For this review, take the finished solid that the model builds, in its own axes (mm). A direction names the side the tool comes from. Coordinates: 2 decimals unless noted, no trailing zeros. Loops run counter-clockwise (first coordinate to the right, second up) from the corner with the lowest first, then second, coordinate; pieces in that order, holes last. Notation, with made-up numbers: (-33.75, -14) - (11.25, -14) arc R21 cw to (11.25, 14) - close; hole circle Ø7 at (0, 20). An arc over 180 degrees is marked (long way). Use one line per item in the form item = value. Start each with the question number.
1. Add section C-C on x = 30. Give the boundary of the cut face in (y, z) (3 decimals).
2. Add section A-A on x = 0. Give the boundary of the cut face in (y, z), and give its area (3 significant figures).
3. Draft analysis for pull direction X (two halves, no side actions). For faces 1 (the face through (39.99, 4.85, 5.58)), 2 (the face through (0, 129, 5)), 3 (the face through (-14.49, 119.24, 5.42)), state which applies: +X half, -X half, draft (parallel to the pull), parting line (faces both ways), or undercut.
4. Machinability: for faces 4 (the face through (-30.163, 4.067, 11.16)), 5 (the face through (43, 44, 5)), 6 (the face through (-33.5, 64, 4)), which of the approach directions +Z, -Z, +X, -X, +Y, -Y give a long, thin tool a straight path to every point of the face, cutting with its end or side? Answer none if there is none.
5. Add section D-D on y = 86. Give the boundary of the cut face in (x, z), and give its area (3 significant figures).
6. Add section B-B on y = 64. Give the boundary of the cut face in (x, z) (3 decimals).
7. For pin 1 Ø4.5 at (x, y) = (30, 67) entering from +Z; pin 2 Ø2 at (x, z) = (24, 7) entering from +Y; pin 3 Ø4 at (y, z) = (101.5, 10) entering from +X, all flat-tipped, find the tip position at first contact; note any pin that passes through.
8. To check wall thickness, follow probe 1 along X at (y, z) = (15.5, 10.5); probe 2 along Y at (x, z) = (-11.5, 4.5); probe 3 along X at (y, z) = (9.5, 7). State the ranges of each line that lie inside material, in increasing order.
```python
from build123d import *

# Parameters (mm, degrees)
SKETCH1_W                                = 86
SKETCH1_H                                = 77
SKETCH1_R                                = 17.5
BOSS_EXTRUDE1_DEPTH                      = 12
CBORE_START                              = 7.62
CBORE_SLOT_FOR_M6_HEX_HEAD_BOLT1_DEPTH   = 4.38
CBORE_SLOT_FOR_M6_HEX_HEAD_BOLT1_2_DEPTH = 7.62
M4X0_7_TAPPED_HOLE1_D                    = 3.3
M4X0_7_TAPPED_HOLE1_DEPTH                = 17.1
M4X0_7_TAPPED_HOLE1_TIP                  = 0.991420021
FILLET1_R                                = 10
CHAMFER1_SIZE                            = 1


# Read off the part's stored shape, not the designer's step: CBORE SLOT for M6 Hex Head Bolt1
with BuildPart() as part:
    # Sketch1 → Boss-Extrude1 (new body)
    # profile 1 of 2: a face of its own
    with BuildSketch(Plane.XY):
        with Locations((0, 40.5)):
            Rectangle(SKETCH1_W, SKETCH1_H)
    # profile 2 of 2: a face of its own
    with BuildSketch(Plane.XY):
        Polygon((-27.043146614, 122.240902798), (-43, 79), (43, 79), (27.043146614, 122.240902798), (24.548889647, 129), (-24.548889647, 129), align=None)
        with Locations((0, 106)):
            Circle(SKETCH1_R, mode=Mode.SUBTRACT)
    extrude(amount=BOSS_EXTRUDE1_DEPTH)

    # CBORE SLOT for M6 Hex Head Bolt1 outline → CBORE SLOT for M6 Hex Head Bolt1 (cut)
    with BuildSketch(Plane.XY.offset(CBORE_START)):
        with BuildLine():
            Line((-22.725, 11.5), (-22.725, 14.5))
            ThreePointArc((-22.725, 14.5), (-30, 21.775), (-37.275, 14.5))
            Line((-37.275, 14.5), (-37.275, 11.5))
            ThreePointArc((-37.275, 11.5), (-30, 4.225), (-22.725, 11.5))
        make_face()
        with BuildLine():
            ThreePointArc((-22.725, 65.5), (-30, 72.775), (-37.275, 65.5))
            Line((-37.275, 65.5), (-37.275, 62.5))
            ThreePointArc((-37.275, 62.5), (-30, 55.225), (-22.725, 62.5))
            Line((-22.725, 62.5), (-22.725, 65.5))
        make_face()
        with BuildLine():
            Line((37.275, 11.5), (37.275, 14.5))
            ThreePointArc((37.275, 14.5), (30, 21.775), (22.725, 14.5))
            Line((22.725, 14.5), (22.725, 11.5))
            ThreePointArc((22.725, 11.5), (30, 4.225), (37.275, 11.5))
        make_face()
        with BuildLine():
            ThreePointArc((37.275, 65.5), (30, 72.775), (22.725, 65.5))
            Line((22.725, 65.5), (22.725, 62.5))
            ThreePointArc((22.725, 62.5), (30, 55.225), (37.275, 62.5))
            Line((37.275, 62.5), (37.275, 65.5))
        make_face()
    extrude(amount=CBORE_SLOT_FOR_M6_HEX_HEAD_BOLT1_DEPTH, mode=Mode.SUBTRACT)

    # CBORE SLOT for M6 Hex Head Bolt1 2 outli → CBORE SLOT for M6 Hex Head Bolt1 2 (cut)
    with BuildSketch(Plane.XY):
        with BuildLine():
            Line((-26.5, 11.5), (-26.5, 14.5))
            ThreePointArc((-26.5, 14.5), (-30, 18), (-33.5, 14.5))
            Line((-33.5, 14.5), (-33.5, 11.5))
            ThreePointArc((-33.5, 11.5), (-30, 8), (-26.5, 11.5))
        make_face()
        with BuildLine():
            ThreePointArc((-33.5, 62.5), (-30, 59), (-26.5, 62.5))
            Line((-26.5, 62.5), (-26.5, 65.5))
            ThreePointArc((-26.5, 65.5), (-30, 69), (-33.5, 65.5))
            Line((-33.5, 65.5), (-33.5, 62.5))
        make_face()
        with BuildLine():
            Line((33.5, 11.5), (33.5, 14.5))
            ThreePointArc((33.5, 14.5), (30, 18), (26.5, 14.5))
            Line((26.5, 14.5), (26.5, 11.5))
            ThreePointArc((26.5, 11.5), (30, 8), (33.5, 11.5))
        make_face()
        with BuildLine():
            ThreePointArc((33.5, 65.5), (30, 69), (26.5, 65.5))
            Line((26.5, 65.5), (26.5, 62.5))
            ThreePointArc((26.5, 62.5), (30, 59), (33.5, 62.5))
            Line((33.5, 62.5), (33.5, 65.5))
        make_face()
    extrude(amount=CBORE_SLOT_FOR_M6_HEX_HEAD_BOLT1_2_DEPTH, mode=Mode.SUBTRACT)

    # M4x0.7 Tapped Hole1
    with Locations(Plane(origin=(-14.849242405, 120.849242405, 12), x_dir=(1, 0, 0), z_dir=(0, 0, 1))):
        with Locations((0, 0), (29.69848481, 0), (29.69848481, -29.69848481), (0, -29.69848481)):
            Hole(M4X0_7_TAPPED_HOLE1_D / 2, depth=M4X0_7_TAPPED_HOLE1_DEPTH)
            with Locations((0, 0, -(M4X0_7_TAPPED_HOLE1_DEPTH + M4X0_7_TAPPED_HOLE1_TIP / 2))):  # 118° drill point
                Cone(0, M4X0_7_TAPPED_HOLE1_D / 2, M4X0_7_TAPPED_HOLE1_TIP, mode=Mode.SUBTRACT)

    # Fillet1
    fillet1_edges = [part.edges().sort_by_distance(p)[0] for p in [
        (-24.548889647, 129, 6),
        (24.548889647, 129, 6),
        (43, 79, 6),
        (43, 2, 6),
        (-43, 2, 6),
        (-43, 79, 6),
    ]]
    fillet(fillet1_edges, radius=FILLET1_R)

    # Chamfer1
    # the kernel refuses this chamfer: 1 mm, written as the material it takes off along each edge
    with BuildSketch(Plane(origin=(-22.725, 62.5, 12), x_dir=(0.9996219169112968, 0, 0.027495876610585647), z_dir=(0, 1, 0)), Plane(origin=(-37.275, 65.5, 12), x_dir=(-0.9996219169112968, 0, 0.02749587661058555), z_dir=(0, -1, 0)), Plane(origin=(-22.725, 11.5, 12), x_dir=(0.9996219169112968, 0, 0.027495876610585647), z_dir=(0, 1, 0)), Plane(origin=(-37.275, 14.5, 12), x_dir=(-0.9996219169112968, 0, 0.02749587661058555), z_dir=(0, -1, 0)), Plane(origin=(37.275, 11.5, 12), x_dir=(0.9996219169112968, 0, 0.02749587661058555), z_dir=(0, 1, 0)), Plane(origin=(22.725, 14.5, 12), x_dir=(-0.9996219169112968, 0, 0.027495876610585647), z_dir=(0, -1, 0)), Plane(origin=(37.275, 62.5, 12), x_dir=(0.9996219169112968, 0, 0.02749587661058555), z_dir=(0, 1, 0)), Plane(origin=(22.725, 65.5, 12), x_dir=(-0.9996219169112968, 0, 0.027495876610585647), z_dir=(0, -1, 0))) as chamfer1_piece_1:
        Polygon((CHAMFER1_SIZE * 0.999621916911, CHAMFER1_SIZE * 0.0274958766106), (-CHAMFER1_SIZE * 0.0274958766106, CHAMFER1_SIZE * 0.999621916911), (0, 0), align=None)
    extrude(amount=3, mode=Mode.SUBTRACT)
    with BuildSketch(Plane(origin=(-30, 65.5, 12), x_dir=(1, 0, 0), z_dir=(0, -1, 0))) as chamfer1_piece_2:
        Polygon((7.275 + CHAMFER1_SIZE, 0), (7.275, -CHAMFER1_SIZE), (7.275, 0), align=None)
    revolve(axis=Axis((-30, 65.5, 12), (0, 0, 1)), revolution_arc=180, mode=Mode.SUBTRACT)
    with BuildSketch(Plane(origin=(-30, 62.5, 12), x_dir=(-1, 0, 0), z_dir=(0, 1, 0))) as chamfer1_piece_3:
        Polygon((7.275 + CHAMFER1_SIZE, 0), (7.275, -CHAMFER1_SIZE), (7.275, 0), align=None)
    revolve(axis=Axis((-30, 62.5, 12), (0, 0, 1)), revolution_arc=180, mode=Mode.SUBTRACT)
    with BuildSketch(Plane(origin=(-14.849242405, 91.150757595, 12), x_dir=(-1, 0, 0), z_dir=(0, -1, 0))) as chamfer1_piece_4:
        Polygon((1.65 + CHAMFER1_SIZE, 0), (1.65, CHAMFER1_SIZE), (1.65, 0), align=None)
    revolve(axis=Axis((-14.849242405, 91.150757595, 12), (0, 0, -1)), mode=Mode.SUBTRACT)
    with BuildSketch(Plane(origin=(14.849242405, 91.150757595, 12), x_dir=(-1, 0, 0), z_dir=(0, -1, 0))) as chamfer1_piece_5:
        Polygon((1.65 + CHAMFER1_SIZE, 0), (1.65, CHAMFER1_SIZE), (1.65, 0), align=None)
    revolve(axis=Axis((14.849242405, 91.150757595, 12), (0, 0, -1)), mode=Mode.SUBTRACT)
    with BuildSketch(Plane(origin=(14.849242405, 120.849242405, 12), x_dir=(-1, 0, 0), z_dir=(0, -1, 0))) as chamfer1_piece_6:
        Polygon((1.65 + CHAMFER1_SIZE, 0), (1.65, CHAMFER1_SIZE), (1.65, 0), align=None)
    revolve(axis=Axis((14.849242405, 120.849242405, 12), (0, 0, -1)), mode=Mode.SUBTRACT)
    with BuildSketch(Plane(origin=(-14.849242405, 120.849242405, 12), x_dir=(-1, 0, 0), z_dir=(0, -1, 0))) as chamfer1_piece_7:
        Polygon((1.65 + CHAMFER1_SIZE, 0), (1.65, CHAMFER1_SIZE), (1.65, 0), align=None)
    revolve(axis=Axis((-14.849242405, 120.849242405, 12), (0, 0, -1)), mode=Mode.SUBTRACT)
    with BuildSketch(Plane(origin=(-33, 2, 12), x_dir=(0, 0.9996219169112968, 0.027495876610585623), z_dir=(1, 0, 0))) as chamfer1_piece_8:
        Polygon((CHAMFER1_SIZE * 0.999621916911, -CHAMFER1_SIZE * 0.0274958766106), (-CHAMFER1_SIZE * 0.0274958766106, -CHAMFER1_SIZE * 0.999621916911), (0, 0), align=None)
    extrude(amount=66, mode=Mode.SUBTRACT)
    with BuildSketch(Plane(origin=(-43, 77.213760058, 12), x_dir=(-0.0274958766105891, 0, -0.9996219169112968), z_dir=(0, -1, 0))) as chamfer1_piece_9:
        Polygon((CHAMFER1_SIZE * 0.999621916911, CHAMFER1_SIZE * 0.0274958766106), (-CHAMFER1_SIZE * 0.0274958766106, CHAMFER1_SIZE * 0.999621916911), (0, 0), align=None)
    extrude(amount=65.213760058, mode=Mode.SUBTRACT)
    with BuildSketch(Plane(origin=(-42.381600361, 80.675778929, 12), x_dir=(0.9378053336703238, -0.3460709940299939, 0.0274958766105856), z_dir=(0.34620188710878685, 0.938160036114476, 0)), Plane(origin=(26.961549873, 122.462018871, 12), x_dir=(-0.9378053336703737, -0.3460709940298588, 0.027495876610585664), z_dir=(0.34620188710865174, -0.9381600361145258, 0))) as chamfer1_piece_10:
        Polygon((CHAMFER1_SIZE * 0.999621916911, CHAMFER1_SIZE * 0.0274958766106), (-CHAMFER1_SIZE * 0.0274958766106, CHAMFER1_SIZE * 0.999621916911), (0, 0), align=None)
    extrude(amount=44.540630952, mode=Mode.SUBTRACT)
    with BuildSketch(Plane(origin=(43, 12, 12), x_dir=(-0.9996219169112968, 0, 0.02749587661058555), z_dir=(0, 1, 0))) as chamfer1_piece_11:
        Polygon((CHAMFER1_SIZE * 0.999621916911, -CHAMFER1_SIZE * 0.0274958766106), (-CHAMFER1_SIZE * 0.0274958766106, -CHAMFER1_SIZE * 0.999621916911), (0, 0), align=None)
    extrude(amount=65.213760058, mode=Mode.SUBTRACT)
    with BuildSketch(Plane(origin=(17.579949511, 129, 12), x_dir=(0, -0.9996219169112968, 0.02749587661058574), z_dir=(-1, 0, 0))) as chamfer1_piece_12:
        Polygon((CHAMFER1_SIZE * 0.999621916911, -CHAMFER1_SIZE * 0.0274958766106), (-CHAMFER1_SIZE * 0.0274958766106, -CHAMFER1_SIZE * 0.999621916911), (0, 0), align=None)
    extrude(amount=35.159899023, mode=Mode.SUBTRACT)
    with BuildSketch(Plane(origin=(17.579949511, 119, 12), x_dir=(0, 1, 0), z_dir=(-1, 0, 0))) as chamfer1_piece_13:
        Polygon((10 - CHAMFER1_SIZE, 0), (10, CHAMFER1_SIZE), (10, 0), align=None)
    revolve(axis=Axis((17.579949511, 119, 12), (0, 0, -1)), revolution_arc=69.744819304, mode=Mode.SUBTRACT)
    with BuildSketch(Plane(origin=(-17.579949511, 119, 12), x_dir=(-0.9381600361144766, 0.34620188710878497, 0), z_dir=(-0.34620188710878497, -0.9381600361144766, 0))) as chamfer1_piece_14:
        Polygon((10 - CHAMFER1_SIZE, 0), (10, CHAMFER1_SIZE), (10, 0), align=None)
    revolve(axis=Axis((-17.579949511, 119, 12), (0, 0, -1)), revolution_arc=69.744819304, mode=Mode.SUBTRACT)
    with BuildSketch(Plane(origin=(-33, 77.213760058, 12), x_dir=(-1, 0, 0), z_dir=(0, -1, 0))) as chamfer1_piece_15:
        Polygon((10, CHAMFER1_SIZE), (10 - CHAMFER1_SIZE, 0), (10, 0), align=None)
    revolve(axis=Axis((-33, 77.213760058, 12), (0, 0, -1)), revolution_arc=20.255180696, mode=Mode.SUBTRACT)
    with BuildSketch(Plane(origin=(33, 77.213760058, 12), x_dir=(1, 0, 0), z_dir=(0, -1, 0))) as chamfer1_piece_16:
        Polygon((10 - CHAMFER1_SIZE, 0), (10, -CHAMFER1_SIZE), (10, 0), align=None)
    revolve(axis=Axis((33, 77.213760058, 12), (0, 0, 1)), revolution_arc=20.255180696, mode=Mode.SUBTRACT)
    with BuildSketch(Plane(origin=(33, 12, 12), x_dir=(0, -1, 0), z_dir=(-1, 0, 0))) as chamfer1_piece_17:
        Polygon((10 - CHAMFER1_SIZE, 0), (10, -CHAMFER1_SIZE), (10, 0), align=None)
    revolve(axis=Axis((33, 12, 12), (0, 0, 1)), revolution_arc=90, mode=Mode.SUBTRACT)
    with BuildSketch(Plane(origin=(-33, 12, 12), x_dir=(-1, 0, 0), z_dir=(0, 1, 0))) as chamfer1_piece_18:
        Polygon((10, -CHAMFER1_SIZE), (10 - CHAMFER1_SIZE, 0), (10, 0), align=None)
    revolve(axis=Axis((-33, 12, 12), (0, 0, 1)), revolution_arc=90, mode=Mode.SUBTRACT)
    with BuildSketch(Plane(origin=(-30, 14.5, 12), x_dir=(1, 0, 0), z_dir=(0, -1, 0))) as chamfer1_piece_19:
        Polygon((7.275 + CHAMFER1_SIZE, 0), (7.275, -CHAMFER1_SIZE), (7.275, 0), align=None)
    revolve(axis=Axis((-30, 14.5, 12), (0, 0, 1)), revolution_arc=180, mode=Mode.SUBTRACT)
    with BuildSketch(Plane(origin=(-30, 11.5, 12), x_dir=(-1, 0, 0), z_dir=(0, 1, 0))) as chamfer1_piece_20:
        Polygon((7.275 + CHAMFER1_SIZE, 0), (7.275, -CHAMFER1_SIZE), (7.275, 0), align=None)
    revolve(axis=Axis((-30, 11.5, 12), (0, 0, 1)), revolution_arc=180, mode=Mode.SUBTRACT)
    with BuildSketch(Plane(origin=(30, 14.5, 12), x_dir=(1, 0, 0), z_dir=(0, -1, 0))) as chamfer1_piece_21:
        Polygon((7.275 + CHAMFER1_SIZE, 0), (7.275, -CHAMFER1_SIZE), (7.275, 0), align=None)
    revolve(axis=Axis((30, 14.5, 12), (0, 0, 1)), revolution_arc=180, mode=Mode.SUBTRACT)
    with BuildSketch(Plane(origin=(30, 11.5, 12), x_dir=(-1, 0, 0), z_dir=(0, 1, 0))) as chamfer1_piece_22:
        Polygon((7.275 + CHAMFER1_SIZE, 0), (7.275, -CHAMFER1_SIZE), (7.275, 0), align=None)
    revolve(axis=Axis((30, 11.5, 12), (0, 0, 1)), revolution_arc=180, mode=Mode.SUBTRACT)
    with BuildSketch(Plane(origin=(0, 106, 12), x_dir=(1, 0, 0), z_dir=(0, -1, 0))) as chamfer1_piece_23:
        Polygon((17.5 + CHAMFER1_SIZE, 0), (17.5, -CHAMFER1_SIZE), (17.5, 0), align=None)
    revolve(axis=Axis((0, 106, 12), (0, 0, 1)), mode=Mode.SUBTRACT)
    with BuildSketch(Plane(origin=(30, 65.5, 12), x_dir=(1, 0, 0), z_dir=(0, -1, 0))) as chamfer1_piece_24:
        Polygon((7.275 + CHAMFER1_SIZE, 0), (7.275, -CHAMFER1_SIZE), (7.275, 0), align=None)
    revolve(axis=Axis((30, 65.5, 12), (0, 0, 1)), revolution_arc=180, mode=Mode.SUBTRACT)
    with BuildSketch(Plane(origin=(30, 62.5, 12), x_dir=(-1, 0, 0), z_dir=(0, 1, 0))) as chamfer1_piece_25:
        Polygon((7.275 + CHAMFER1_SIZE, 0), (7.275, -CHAMFER1_SIZE), (7.275, 0), align=None)
    revolve(axis=Axis((30, 62.5, 12), (0, 0, 1)), revolution_arc=180, mode=Mode.SUBTRACT)


solid = part.part
```
Conclusion:
q1.outline = (2, 0) - (8, 0) - (8, 7.62) - (4.225, 7.62) - (4.225, 11) - (3.225, 12) - (3, 12) - (2, 11) - close; (18, 0) - (59, 0) - (59, 7.62) - (55.225, 7.62) - (55.225, 11) - (54.225, 12) - (22.775, 12) - (21.775, 11) - (21.775, 7.62) - (18, 7.62) - close; (69, 0) - (114.228, 0) - (114.228, 11) - (111.34, 12) - (73.775, 12) - (72.775, 11) - (72.775, 7.62) - (69, 7.62) - close
q2.outline = (2, 0) - (88.5, 0) - (88.5, 11) - (87.5, 12) - (3, 12) - (2, 11) - close; (123.5, 0) - (129, 0) - (129, 11) - (128, 12) - (124.5, 12) - (123.5, 11) - close
q2.area = 1,100 mm^2
q3.face_1 = +X half
q3.face_2 = draft
q3.face_3 = undercut
q4.face_4 = +Z
q4.face_5 = +Z, -Z, +X, +Y, -Y
q4.face_6 = +Z, -Z
q5.outline = (-40.42, 0) - (40.42, 0) - (40.42, 11) - (39.35, 12) - (-39.35, 12) - (-40.42, 11) - close
q5.area = 969 mm^2
q6.outline = (-43, 0) - (-33.5, 0) - (-33.5, 7.62) - (-37.275, 7.62) - (-37.275, 11) - (-38.275, 12) - (-42, 12) - (-43, 11) - close; (-26.5, 0) - (26.5, 0) - (26.5, 7.62) - (22.725, 7.62) - (22.725, 11) - (21.725, 12) - (-21.725, 12) - (-22.725, 11) - (-22.725, 7.62) - (-26.5, 7.62) - close; (33.5, 0) - (43, 0) - (43, 11) - (42, 12) - (38.275, 12) - (37.275, 11) - (37.275, 7.62) - (33.5, 7.62) - close
q7.pin_1 = 7.62
q7.pin_2 = 127.4
q7.pin_3 = 35.44
q8.probe_1 = -43 to -37.21, -22.79 to 22.79, 37.21 to 43
q8.probe_2 = 2 to 92.81, 119.19 to 129
q8.probe_3 = -42.68 to -32.87, -27.13 to 27.13, 32.87 to 42.68
